Here's how the part is built. I have some questions about the finished solid (model axes, mm). Coordinates: 2 decimals unless noted, no trailing zeros. Loops run counter-clockwise (first coordinate to the right, second up) from the corner with the lowest first, then second, coordinate; pieces in that order, holes last.
from build123d import *

# Parameters (mm, degrees)
F0_W     = 75.5
F0_H     = 200
F1_DEPTH = 2.5
F2_R     = 3.4
F2_R_2   = 3.5
F2_R_3   = 10
F2_R_4   = 2.75
F3_DEPTH = 5
F4_R     = 3


with BuildPart() as f1:
    # F0 (on Right) → F1 (new body, symmetric)
    with BuildSketch(Plane.YZ):
        Rectangle(F0_W, F0_H)
    extrude(amount=F1_DEPTH, both=True)

    # F2 (on face) → F3 (cut)
    with BuildSketch(Plane.YZ.offset(2.5)):
        with Locations((22.75, 85)):
            Circle(F2_R)
        with Locations((22.75, 55)):
            Circle(F2_R)
        with Locations((22.75, -55)):
            Circle(F2_R)
        with Locations((22.75, -25)):
            Circle(F2_R)
        with Locations((-7.25, 85)):
            Circle(F2_R_2)
        with Locations((-7.25, -55)):
            Circle(F2_R_2)
        with Locations((-22.25, 15)):
            Circle(F2_R_3)
        with Locations((-22.25, 38)):
            Circle(F2_R_4)
        with Locations((-4.25, 38)):
            Circle(F2_R_4)
        with Locations((-22.25, -8)):
            Circle(F2_R_4)
        with Locations((-4.25, -8)):
            Circle(F2_R_4)
    extrude(amount=-F3_DEPTH, mode=Mode.SUBTRACT)

    # F4
    f4_edges = [f1.edges().sort_by_distance(p)[0] for p in [
        (0, 37.75, 100),
    ]]
    fillet(f4_edges, radius=F4_R)


solid = f1.part
Q1. Will this pin go through, and if not, where does the flat tip stop? P1, Ø6, axis at y = 22.75, z = 55, coming from the +X side.
Q2. Suppose I cut it at A-A on z = -25. Write out the boundary of the cut face in (x, y), and give its area (4 significant figures).
Q3. Please list where these lines run through material, in increasing order: probe 1 along Z at (x, y) = (0.5, 22.75); probe 2 along Z at (x, y) = (-0.9, -7.25); probe 3 along Z at (x, y) = (0.95, -4.25).
Q4. We'd pull the mould along Z, two halves only. Please class faces 1 (the cylindrical face through (0.04, -12.71, 18)), 2 (the flat face through (0, -1, -100)), 3 (the flat face through (0, 37.75, -3)): pulls with the +Z half, pulls with the -Z half, needs draft (parallel to the pull), parting line crosses it, or undercut.
Q5. Suppose I cut it at D-D on y = -15.5. Write out the boundary of the cut face in (x, z), and give its area (3 significant figures).
Q6. Suppose I cut it at B-B on z = 38. Write out the boundary of the cut face in (x, y), and give its area (4 significant figures).
Q7. Suppose I cut it at C-C on x = -1.1. State how many separate pieces and enclosed holes the cut face has, and give its area (3 significant figures).
Check values:
1. P1: passes through
2. outline: (-2.5, -37.75) - (2.5, -37.75) - (2.5, 19.35) - (-2.5, 19.35) - close; (-2.5, 26.15) - (2.5, 26.15) - (2.5, 37.75) - (-2.5, 37.75) - close
2. area: 343.5 mm2
3. probe 1: z = -100 to -58.4, -51.6 to -28.4, -21.6 to 51.6, 58.4 to 81.6, 88.4 to 100
3. probe 2: z = -100 to -58.5, -51.5 to 81.5, 88.5 to 100
3. probe 3: z = -100 to -56.8, -53.2 to -10.75, -5.25 to 35.25, 40.75 to 83.2, 86.8 to 100
4. face 1: undercut
4. face 2: pulls with the -Z half
4. face 3: needs draft
5. outline: (-2.5, -100) - (2.5, -100) - (2.5, 7.62) - (-2.5, 7.62) - close; (-2.5, 22.38) - (2.5, 22.38) - (2.5, 100) - (-2.5, 100) - close
5. area: 926 mm2
6. outline: (-2.5, -37.75) - (2.5, -37.75) - (2.5, -25) - (-2.5, -25) - close; (-2.5, -19.5) - (2.5, -19.5) - (2.5, -7) - (-2.5, -7) - close; (-2.5, -1.5) - (2.5, -1.5) - (2.5, 37.75) - (-2.5, 37.75) - close
6. area: 322.5 mm2
7. separate pieces: 1
7. enclosed holes: 11
7. area: 14,500 mm2
